For this review, take the finished solid that the model builds, in its own axes (mm). Give positions to 0.01 mm unless a question says otherwise; leave off trailing zeros. Loops run counter-clockwise (first coordinate to the right, second up) from the corner with the lowest first, then second, coordinate; pieces in that order, holes last.
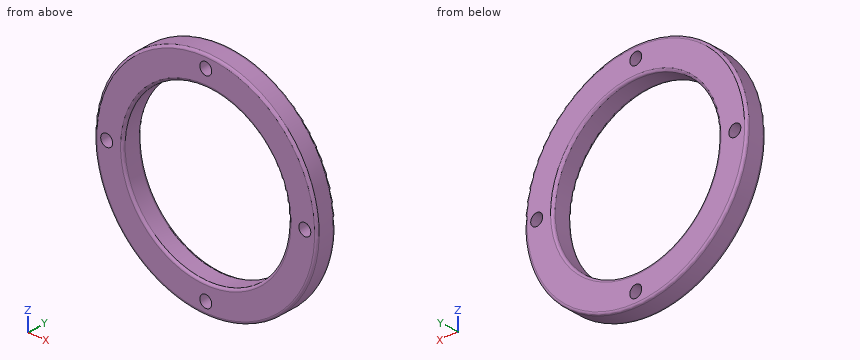
```python
from build123d import *

# Parameters (mm, degrees)
SKETCH1_R           = 46.6
SKETCH1_R_2         = 34.7
SKETCH1_R_3         = 2.5
BOSS_EXTRUDE1_DEPTH = 8.5
FILLET1_R           = 1


with BuildPart() as part:
    # Sketch1 → Boss-Extrude1 (new body)
    with BuildSketch(Plane(origin=(0, 0, 0), x_dir=(1, 0, 0), z_dir=(0, 1, 0))):
        with Locations(Location((0, 0, 0), (0, 0, 270))):
            Circle(SKETCH1_R)
        with Locations(Location((0, 0, 0), (0, 0, 270))):
            Circle(SKETCH1_R_2, mode=Mode.SUBTRACT)
        with Locations(Location((0, 41.5, 0), (0, 0, 270))):
            Circle(SKETCH1_R_3, mode=Mode.SUBTRACT)
        with Locations(Location((41.5, 0, 0), (0, 0, 270))):
            Circle(SKETCH1_R_3, mode=Mode.SUBTRACT)
        with Locations(Location((0, -41.5, 0), (0, 0, 270))):
            Circle(SKETCH1_R_3, mode=Mode.SUBTRACT)
        with Locations(Location((-41.5, 0, 0), (0, 0, 270))):
            Circle(SKETCH1_R_3, mode=Mode.SUBTRACT)
    extrude(amount=BOSS_EXTRUDE1_DEPTH)

    # Fillet1
    fillet1_edges = [part.edges().sort_by_distance(p)[0] for p in [
        (0, 0, -46.6),
        (0, 8.5, -46.6),
        (0, 0, -34.7),
        (0, 8.5, -34.7),
    ]]
    fillet(fillet1_edges, radius=FILLET1_R)


solid = part.part
```
Item 1: Take a section at B-B on x = 0. Give the boundary of the cut face in (y, z).
Answer:
outline: (0, -45.6) arc R1 ccw to (1, -46.6) - (7.5, -46.6) arc R1 ccw to (8.5, -45.6) - (8.5, -44) - (0, -44) - close; (0, -39) - (8.5, -39) - (8.5, -35.7) arc R1 ccw to (7.5, -34.7) - (1, -34.7) arc R1 ccw to (0, -35.7) - close; (0, 35.7) arc R1 ccw to (1, 34.7) - (7.5, 34.7) arc R1 ccw to (8.5, 35.7) - (8.5, 39) - (0, 39) - close; (0, 44) - (8.5, 44) - (8.5, 45.6) arc R1 ccw to (7.5, 46.6) - (1, 46.6) arc R1 ccw to (0, 45.6) - close
Item 2: For L1, parallel to X at y = 6, z = 0; L2, parallel to X at y = 1.75, z = -9; L3, parallel to Z at x = 13.5, y = 7.75, list the stretches that pass through material, from the lowest coordinate up.
Answer:
L1: x = -46.6 to -44, -39 to -34.7, 34.7 to 39, 44 to 46.6
L2: x = -45.72 to -33.51, 33.51 to 45.72
L3: z = -44.57 to -32, 32 to 44.57
Item 3: Take a section at A-A on z = 0. Give the boundary of the cut face in (x, y).
Answer:
outline: (-46.6, 1) arc R1 ccw to (-45.6, 0) - (-44, 0) - (-44, 8.5) - (-45.6, 8.5) arc R1 ccw to (-46.6, 7.5) - close; (-39, 0) - (-35.7, 0) arc R1 ccw to (-34.7, 1) - (-34.7, 7.5) arc R1 ccw to (-35.7, 8.5) - (-39, 8.5) - close; (34.7, 1) arc R1 ccw to (35.7, 0) - (39, 0) - (39, 8.5) - (35.7, 8.5) arc R1 ccw to (34.7, 7.5) - close; (44, 0) - (45.6, 0) arc R1 ccw to (46.6, 1) - (46.6, 7.5) arc R1 ccw to (45.6, 8.5) - (44, 8.5) - close
Item 4: Clearance check with flat-ended pins moving along their axes: pin 1 Ø6 at (x, z) = (-41.5, 0) entering from +Y; pin 2 Ø3 at (y, z) = (3, 15.5) entering from +X; pin 3 Ø5 at (y, z) = (6, -5) entering from -X; pin 4 Ø5 at (y, z) = (1, 19) entering from -X. State where each tip first meets the part, or that it passes through.
Answer:
pin 1: stops at y = 8.5
pin 2: stops at x = 44.45
pin 3: stops at x = -46.53
pin 4: stops at x = -43.58
Item 5: Take a section at C-C on y = 2.5. Give the boundary of the cut face in (x, z).
Answer:
outline: circle Ø93.2 at (0, 0); hole circle Ø5 at (-41.5, 0); hole circle Ø69.4 at (0, 0); hole circle Ø5 at (0, -41.5); hole circle Ø5 at (0, 41.5); hole circle Ø5 at (41.5, 0)
